Geometry check sheet. Reference: the model listing, model coordinates, mm. A direction names the side the tool comes from. Coordinates: 2 decimals unless noted, no trailing zeros. Write each loop counter-clockwise with the first axis right and the second up, starting at its lowest first coordinate (ties: lowest second). Pieces come first, ordered by that corner, then holes. Notation, with made-up numbers: (51.25, -37) -> (107.25, -37) arc R10 cw to (107.25, -19) -> close; hole circle Ø10 at (14, 18). An arc over 180 degrees is marked (long way). Answer in a Markdown table with one row per item. Add a question column.
Q1. Tool access check on faces 4 (the face through (22.225, 13, -69)), 5 (the face through (13, 25.4, -69)). Record the directions out of +Z, -Z, +X, -X, +Y, -Y that give a thin tool (end or side, any length) a straight path to the whole face; none if there is none.
Q2. Gauge pin test, flat end, axial feed: P1, Ø8, axis at x = 6.5, y = 5.5, coming from the +Z side. Record the tip position at first contact, or that the pin passes through.
Q3. Section check B-B, the plane x = 5. Record the boundary of the cut face in (y, z) (3 decimals).
Q4. Section check D-D, the plane x = 12.7. Record the boundary of the cut face in (y, z) (3 decimals).
Q5. Thickness scan on line 1 (X direction, y = 6.5, z = -82) (3 decimals); line 2 (X direction, y = 1.5, z = -127). Record the ranges inside material, lowest first.
Q6. Release check for a two-part mould opening along X. For faces 1 (the face through (13, 0, -69)), 2 (the face through (3.175, 13, -69)), 3 (the face through (0, 13, -69)) record: pulls with the +X half, pulls with the -X half, needs draft (parallel to the pull), parting line crosses it, or undercut.
Q7. Section check A-A, the plane z = -127. Record the boundary of the cut face in (x, y) (3 decimals).
Autodesk Inventor part; units mm, degrees
ref_plane "YZ Plane" through (0, 0, 0) normal (1, 0, 0) x (0, 1, 0)
ref_plane "XZ Plane" through (0, 0, 0) normal (0, 1, 0) x (-1, 0, 0)
ref_plane "XY Plane" through (0, 0, 0) normal (0, 0, 1) x (1, 0, 0)
sketch "Sketch1" plane through (0, 0, 0) normal (0, 0, 1) x (1, 0, 0)
  line L0 (0, 0) -> (25.4, 0)
  line L1 (25.4, 0) -> (25.4, 25.4)
  line L2 (25.4, 25.4) -> (0, 25.4)
  line L3 (0, 25.4) -> (0, 0)
  line L4 (3.175, 3.175) -> (22.225, 3.175)
  line L5 (22.225, 3.175) -> (22.225, 22.225)
  line L6 (22.225, 22.225) -> (3.175, 22.225)
  line L7 (3.175, 22.225) -> (3.175, 3.175)
  dimension "d0" = 25.4
  dimension "d1" = 25.4
  dimension "d2" = 3.175
extrude "Extrusion1" add sketch "Sketch1" against normal blind 139.7
sketch "Sketch2" plane through (0, 25.4, 0) normal (0, 1, 0) x (1, 0, 0)
  line L0 (25.4, 139.7) -> (0, 139.7)
  point P0 (12.7, 127)
  dimension "d5" = 12.7
hole "Hole1" at (12.7, 25.4, -127) direction (0, -1, 0) diameter 12.7 depth 25.4 tip angle 118
properties part number "short thing"
Calculated:
| question | item | result |
|---|---|---|
| 1 | face 4 | +Z, -Z |
| 1 | face 5 | +Z, -Z, +X, -X, +Y |
| 2 | P1 | stops at z = 0 |
| 3 | outline | (0, -139.7) -> (3.175, -139.7) -> (3.175, 0) -> (0, 0) -> close; (22.225, -139.7) -> (25.4, -139.7) -> (25.4, 0) -> (22.225, 0) -> close |
| 4 | outline | (0, -139.7) -> (3.175, -139.7) -> (3.175, -133.35) -> (0, -133.35) -> close; (0, -120.65) -> (3.175, -120.65) -> (3.175, 0) -> (0, 0) -> close; (22.225, -139.7) -> (25.4, -139.7) -> (25.4, -133.35) -> (22.225, -133.35) -> close; (22.225, -120.65) -> (25.4, -120.65) -> (25.4, 0) -> (22.225, 0) -> close |
| 5 | line 1 | x = 0 to 3.175, 22.225 to 25.4 |
| 5 | line 2 | x = 0 to 6.35, 19.05 to 25.4 |
| 6 | face 1 | needs draft |
| 6 | face 2 | undercut |
| 6 | face 3 | pulls with the -X half |
| 7 | outline | (0, 0) -> (6.35, 0) -> (6.35, 3.175) -> (3.175, 3.175) -> (3.175, 22.225) -> (6.35, 22.225) -> (6.35, 25.4) -> (0, 25.4) -> close; (19.05, 0) -> (25.4, 0) -> (25.4, 25.4) -> (19.05, 25.4) -> (19.05, 22.225) -> (22.225, 22.225) -> (22.225, 3.175) -> (19.05, 3.175) -> close |
